Verification items for the finished model (mm, model axes). Give positions to 0.01 mm unless a question says otherwise; leave off trailing zeros. Loops run counter-clockwise (first coordinate to the right, second up) from the corner with the lowest first, then second, coordinate; pieces in that order, holes last. Notation, with made-up numbers: (11.25, 26.25) - (32.25, 26.25) arc R32 cw to (32.25, 58.25) - close; hole circle Ø2 at (8, 33.5). An arc over 180 degrees is marked (long way). Answer in a Markdown table with one row per item.
Autodesk Inventor part; units mm, degrees
ref_plane "YZ Plane" through (0, 0, 0) normal (1, 0, 0) x (0, 1, 0)
ref_plane "XZ Plane" through (0, 0, 0) normal (0, 1, 0) x (-1, 0, 0)
ref_plane "XY Plane" through (0, 0, 0) normal (0, 0, 1) x (1, 0, 0)
sketch "Sketch1" plane through (0, 0, 0) normal (1, 0, 0) x (0, 1, 0)
  circle A0 centre (0, 0) radius 1.5
  line L0 (-7.5, 17.5) -> (-7.5, -17.5)
  line L1 (-7.5, -17.5) -> (7.5, -17.5)
  line L2 (7.5, -17.5) -> (7.5, 17.5)
  line L3 (7.5, 17.5) -> (-7.5, 17.5)
  line L4 (-7.5, 17.5) -> (7.5, -17.5) construction
  line L5 (-7.5, -17.5) -> (7.5, 17.5) construction
  dimension "d0" = 3
  dimension "d1" = 35
  dimension "d2" = 15
extrude "Extrusion1" add sketch "Sketch1" along normal blind 3
fillet "Fillet1" radius 2 4 edges at (1.5, 7.5, 17.5) (1.5, -7.5, 17.5) (1.5, -7.5, -17.5) (1.5, 7.5, -17.5)
properties part number "Plate"
Q1. Sectioned sample at C-C (z = 0). Record the cut outline in (x, y).
Completed:
| item | result |
|---|---|
| outline | (0, -7.5) - (3, -7.5) - (3, -1.5) - (0, -1.5) - close; (0, 1.5) - (3, 1.5) - (3, 7.5) - (0, 7.5) - close |
Q2. Draft check along Y on faces 1 (the face through (1, 0, 17.5)), 2 (the face through (1.48, -1.5, -0.07)), 3 (the face through (1.52, 6.9, -16.93)). Enter one of: +Y half, -Y half, draft (parallel to the pull), parting line (faces both ways), or undercut.
Completed:
| item | result |
|---|---|
| face 1 | draft |
| face 2 | undercut |
| face 3 | +Y half |
Q3. Thickness scan on line 1 (Z direction, x = 0.75, y = 0); line 2 (Y direction, x = 2.75, z = -0.5); line 3 (Z direction, x = 1.65, y = -6). Record the ranges inside material, lowest first.
Completed:
| item | result |
|---|---|
| line 1 | -17.5 to -1.5, 1.5 to 17.5 |
| line 2 | -7.5 to -1.41, 1.41 to 7.5 |
| line 3 | -17.44 to 17.44 |
Q4. Go/stop test with a flat-tipped pin: P1, Ø1.8, axis at y = 0, z = 0, coming from the -X side. Record where the tip stops, or that it passes through.
Completed:
| item | result |
|---|---|
| P1 | through |
Q5. Sectioned sample at B-B (y = 0). Record the cut outline in (x, z), and give its area (3 significant figures).
Completed:
| item | result |
|---|---|
| outline | (0, -17.5) - (3, -17.5) - (3, -1.5) - (0, -1.5) - close; (0, 1.5) - (3, 1.5) - (3, 17.5) - (0, 17.5) - close |
| area | 96.0 mm^2 |
Q6. Sectioned sample at A-A (x = 1.4). Record the cut outline in (y, z), and give its area (3 significant figures).
Completed:
| item | result |
|---|---|
| outline | (-7.5, -15.5) arc R2 ccw to (-5.5, -17.5) - (5.5, -17.5) arc R2 ccw to (7.5, -15.5) - (7.5, 15.5) arc R2 ccw to (5.5, 17.5) - (-5.5, 17.5) arc R2 ccw to (-7.5, 15.5) - close; hole circle Ø3 at (0, 0) |
| area | 514 mm^2 |
